For this review, take the finished solid that the model builds, in its own axes (mm). Face numbers are marked on the shaded views. A direction names the side the tool comes from. Round coordinates to 2 decimals unless told otherwise and drop trailing zeros. Order: outer loops, then holes, each group sorted by start corner. A loop starts at its lowest first (then second) coordinate and runs counter-clockwise, first axis right, second up. Notation, with made-up numbers: M -23,-11.75 L 28,-11.75 A29 ccw 28,10.25 Z; hole C 31.25,87.5 d7. An arc over 180 degrees is marked long. Put each result on its own line as item: value.
Autodesk Inventor part; units mm, degrees
ref_plane "YZ Plane" through (0, 0, 0) normal (1, 0, 0) x (0, 1, 0)
ref_plane "XZ Plane" through (0, 0, 0) normal (0, 1, 0) x (-1, 0, 0)
ref_plane "XY Plane" through (0, 0, 0) normal (0, 0, 1) x (1, 0, 0)
sketch "Sketch1" plane through (0, 0, 0) normal (0, 0, 1) x (1, 0, 0)
  line L0 (-26, 0) -> (-35.5, 0)
  circle A0 centre (-35.5, 0) radius 5
  line L1 (0, 0) -> (0, 5.7402)
  arc A1 (-40.3169, 8.1883) -> (-40.3169, -8.1883) centre (-35.5, 0) ccw
  line L2 (-40.3169, 8.1883) -> (-13.9437, 23.7028)
  line L3 (-40.3169, -8.1883) -> (-13.9437, -23.7028)
  arc A2 (-13.9437, -23.7028) -> (0, -27.5) centre (0, 0) ccw
  arc A3 (0, 27.5) -> (-13.9437, 23.7028) centre (0, 0) ccw
  line L4 (26, 0) -> (35.5, 0)
  circle A4 centre (35.5, 0) radius 5
  arc A5 (40.3169, -8.1883) -> (40.3169, 8.1883) centre (35.5, 0) ccw
  line L5 (40.3169, 8.1883) -> (13.9437, 23.7028)
  line L6 (40.3169, -8.1883) -> (13.9437, -23.7028)
  arc A6 (0, -27.5) -> (13.9437, -23.7028) centre (0, 0) ccw
  arc A7 (13.9437, 23.7028) -> (0, 27.5) centre (0, 0) ccw
  dimension "d1" = 35.5
  dimension "d2" = 10
  dimension "d15" = 19
extrude "Extrusion1" add sketch "Sketch1" along normal blind 8
sketch "Sketch2" plane through (0, 0, 8) normal (0, 0, 1) x (1, 0, 0)
  circle A0 centre (0, 0) radius 26.5
  dimension "d6" = 53
extrude "Extrusion2" add sketch "Sketch2" along normal blind 8
sketch "Sketch3" plane through (0, 0, 16) normal (0, 0, 1) x (1, 0, 0)
  circle A0 centre (0, 0) radius 10
  circle A1 centre (0, 0) radius 12.5
  dimension "d9" = 20
  dimension "d10" = 25
extrude "Extrusion3" add sketch "Sketch3" along normal blind 5
sketch "Sketch4" plane through (0, 0, 16) normal (0, 0, 1) x (1, 0, 0)
  circle A0 centre (0, 0) radius 10
extrude "Extrusion4" cut sketch "Sketch4" against normal blind 30
properties part number "RODAMIENTO DE PARED"
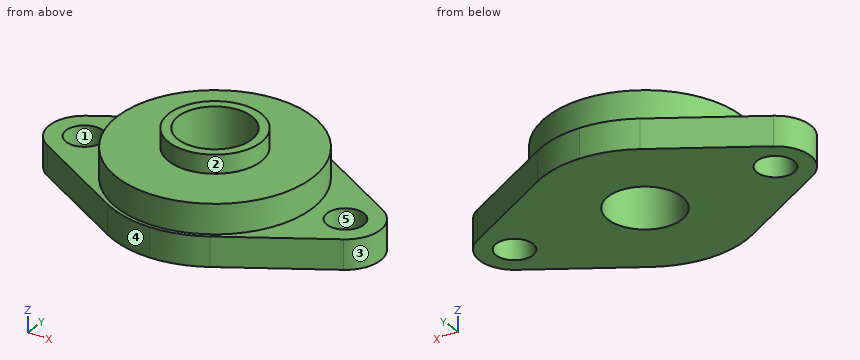
(1) For the marked faces 1 and 2, list the 3-axis set-ups (+Z, -Z, +X, -X, +Y, -Y) from which the entire face can be reached by the end or side of a thin tool; tool diameter is ignored.
A:
face 1: +Z, -Z
face 2: +Z
(2) Add section A-A on z = 4. Give the boundary of the cut face in (x, y).
A:
outline: M -40.32,-8.19 L -13.94,-23.7 A27.5 ccw 0,-27.5 A27.5 ccw 13.94,-23.7 L 40.32,-8.19 A9.5 ccw 40.32,8.19 L 13.94,23.7 A27.5 ccw 0,27.5 A27.5 ccw -13.94,23.7 L -40.32,8.19 A9.5 ccw Z; hole C -35.5,0 d10; hole C 0,0 d20; hole C 35.5,0 d10
(3) Add section C-C on x = 36.5. Give the boundary of the cut face in (y, z).
A:
outline: M -10.43,0 L -4.9,0 L -4.9,8 L -10.43,8 Z; M 4.9,0 L 10.43,0 L 10.43,8 L 4.9,8 Z
(4) Insertion check: pin 1 Ø9 at (x, y) = (-35.5, 0) entering from +Z; pin 2 Ø10 at (y, z) = (-19.5, 16) entering from -X; pin 3 Ø1.5 at (x, y) = (-22, -12) entering from +Z; pin 4 Ø1.5 at (x, z) = (10, 7) entering from -Y. Each pin has a flat end and moves straight along its axis. Give the tip position at first contact, or say it passes through.
A:
pin 1: passes through
pin 2: stops at x = -22.18
pin 3: stops at z = 16
pin 4: stops at y = -25.9
(5) Add section D-D on y = -19.5. Give the boundary of the cut face in (x, z).
A:
outline: M -21.09,0 L 21.09,0 L 21.09,8 L 17.94,8 L 17.94,16 L -17.94,16 L -17.94,8 L -21.09,8 Z
(6) To check wall thickness, follow L1, parallel to Y at x = 0.5, z = 5.5; L2, parallel to Y at x = 0, z = 12.25; L3, parallel to Z at x = -20.5, y = 2.5. State the ranges of each line that lie inside material, in increasing order.
A:
L1: y = -27.5 to -9.99, 9.99 to 27.5
L2: y = -26.5 to -10, 10 to 26.5
L3: z = 0 to 16
(7) Add section B-B on y = 0. Give the boundary of the cut face in (x, z), then the cut area to 3 significant figures.
A:
outline: M -45,0 L -40.5,0 L -40.5,8 L -45,8 Z; M -30.5,0 L -10,0 L -10,21 L -12.5,21 L -12.5,16 L -26.5,16 L -26.5,8 L -30.5,8 Z; M 10,0 L 30.5,0 L 30.5,8 L 26.5,8 L 26.5,16 L 12.5,16 L 12.5,21 L 10,21 Z; M 40.5,0 L 45,0 L 45,8 L 40.5,8 Z
area: 689 mm2
(8) Draft analysis for pull direction X (two halves, no side actions). For the marked faces 3, 4 and 5, state which applies: released by +X, released by -X, zero draft, split by the parting line, or undercut.
A:
face 3: released by +X
face 4: released by -X
face 5: undercut
